Can you work these out from the drawing? Everything is in mm from the part's minimum corner. A direction names the side the tool comes from. Coordinates: 2 decimals unless noted, no trailing zeros. Loops run counter-clockwise (first coordinate to the right, second up) from the corner with the lowest first, then second, coordinate; pieces in that order, holes last. Notation, with made-up numbers: (28.25, 9) -> (80.25, 9) arc R19 cw to (80.25, 40) -> close; hole circle Ø6 at (-29.5, 55.25). An arc over 180 degrees is marked (long way). One line per question, with ' | ' between items.
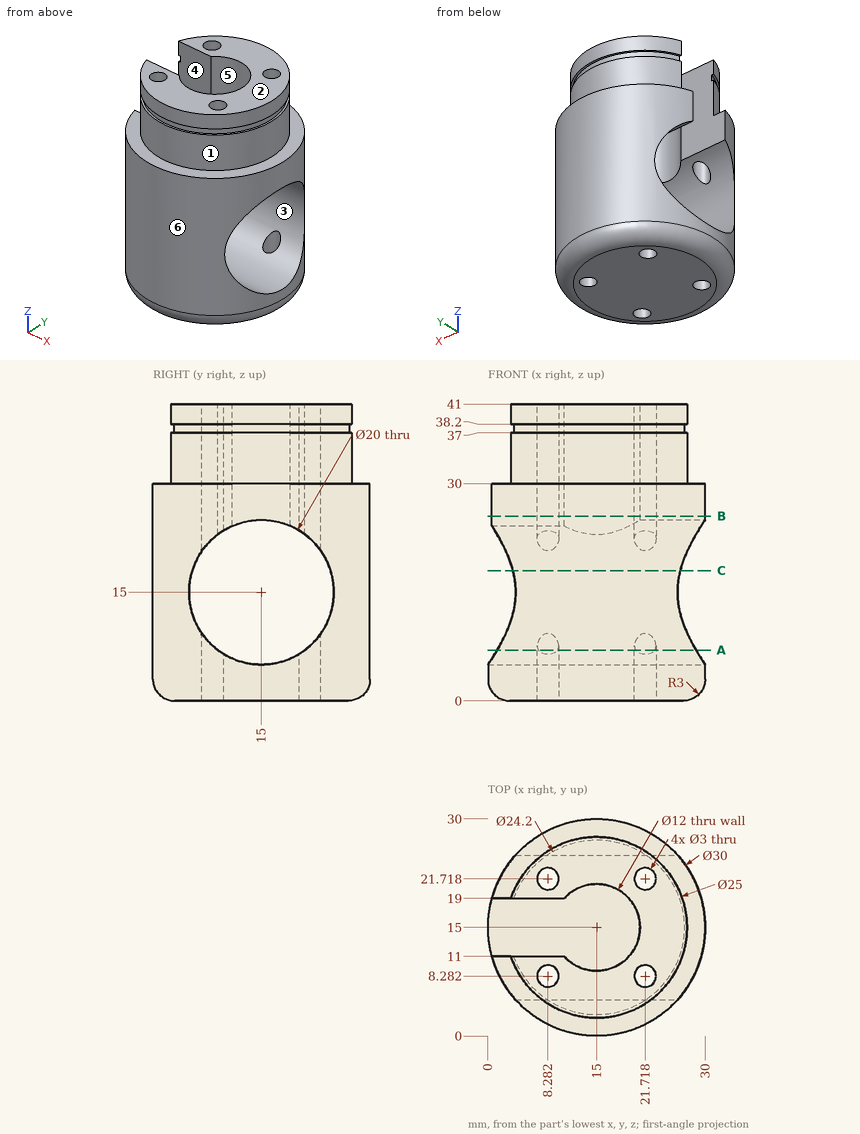
Q1. Imagine slicing it at A-A on z = 7. Write out the boundary of the cut face in (x, y) (1 decimal), plus the area to 3 significant figures.
Values follow:
outline: (1.3, 9) arc R15 ccw to (28.7, 9) -> (23, 9) arc R1.5 cw (long way) to (20.4, 9) -> (9.6, 9) arc R1.5 cw (long way) to (7, 9) -> close; (1.3, 21) -> (7, 21) arc R1.5 cw (long way) to (9.6, 21) -> (20.4, 21) arc R1.5 cw (long way) to (23, 21) -> (28.7, 21) arc R15 ccw to start | area: 334 mm2
Q2. We'd pull the mould along Y, two halves only. Please class the marked faces 1, 2 and 3: released by +Y, released by -Y, zero draft, split by the parting line, or undercut.
Values follow:
face 1: split by the parting line | face 2: zero draft | face 3: undercut
Q3. For pin 1 (8 mm diameter, centred on x = 6.5, z = 30, fed in from -Y); pin 2 (9.5 mm diameter, centred on x = 15, y = 15, fed in from +Z); pin 3 (4 mm diameter, centred on y = 3, z = 18.5, fed in from -X), each with a flat end and sliding along its axis, tell me the tip position at first contact or that it passes through.
Values follow:
pin 1: stops at y = 0.69 | pin 2: stops at z = 6.2 | pin 3: stops at x = 3.82
Q4. For the marked faces 4, 5 and 6, which set-ups out of +Z, -Z, +X, -X, +Y, -Y let a thin tool reach every point of the face, with its end or its side?
Values follow:
face 4: +Z, -X | face 5: +Z | face 6: +Z, -Z
Q5. Please list where these lines run through material, in increasing order: L1, parallel to Y at x = 15, z = 28.5; L2, parallel to Y at x = 9, z = 26.5 (1 decimal); L3, parallel to Y at x = 20, z = 32 (1 decimal). Write a range as [from, to].
Values follow:
L1: y = [0, 9], [21, 30] | L2: y = [1.3, 7], [9.6, 11], [19, 20.4], [23, 28.7] | L3: y = [3.5, 11.7], [18.3, 26.5]
Q6. Imagine slicing it at B-B on z = 25.5. Write out the boundary of the cut face in (x, y), plus the area to 3 significant figures.
Values follow:
outline: (0.54, 11) arc R15 ccw (long way) to (0.54, 19) -> (10.53, 19) arc R6 cw (long way) to (10.53, 11) -> close; hole circle Ø3 at (8.28, 8.28); hole circle Ø3 at (8.28, 21.72); hole circle Ø3 at (21.72, 8.28); hole circle Ø3 at (21.72, 21.72) | area: 491 mm2
Q7. Imagine slicing it at C-C on z = 18. Write out the boundary of the cut face in (x, y) (1 decimal).
Values follow:
outline: (3.4, 5.5) arc R15 ccw to (26.6, 5.5) -> close; (3.4, 24.5) -> (26.6, 24.5) arc R15 ccw to start
